CAD build for the part. Positions are in the model's coordinates, mm. Round coordinates to 2 decimals unless told otherwise and drop trailing zeros. Order: outer loops, then holes, each group sorted by start corner. A loop starts at its lowest first (then second) coordinate and runs counter-clockwise, first axis right, second up. Notation, with made-up numbers: (82.5, -11) -> (117.5, -11) arc R24 ccw to (117.5, 25) -> close; hole circle Ø8 at (23.5, 77). An arc over 180 degrees is marked (long way). Return JSON: item names as keys, results as strings. Group by question number.
Q1. Flat gauge pins, fed straight in: pin 1 (4 mm diameter, centred on y = -3, z = -8, fed in from +X); pin 2 (5 mm diameter, centred on y = -1, z = 7, fed in from -X); pin 3 (8 mm diameter, centred on y = -2, z = -3, fed in from +X). Where does each tip first touch, or does it go through?
Q2. Cut at C-C (x = 439). Write the cut outline in (y, z), then the cut area to 3 significant figures.
Q3. Cut at A-A (y = 3.5). Write the cut outline in (x, z), then the cut area to 3 significant figures.
Q4. Probe line 1 along Y through (x, z) = (187.5, -6.75); line 2 along X through (y, z) = (9.25, -2.5). List the from-to ranges inside material, lowest first.
Q5. Cut at B-B (z = -1.75). Write the cut outline in (x, y), then the cut area to 3 significant figures.
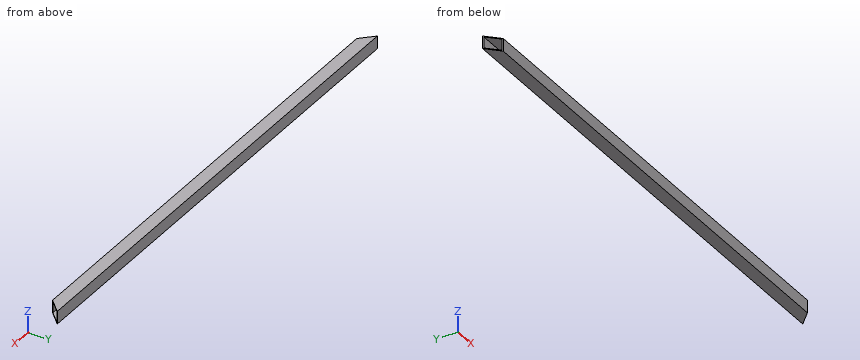
from build123d import *

# Parameters (mm, degrees)
SKETCH1_W               = 20
SKETCH1_H               = 20
SKETCH1_W_2             = 17.6
SKETCH1_H_2             = 17.6
BOSS_EXTRUDE1_DEPTH     = 800
CUT_EXTRUDE1_DEPTH      = 1
CUT_EXTRUDE1_DEPTH_BACK = 21
CUT_EXTRUDE2_DEPTH      = 1
CUT_EXTRUDE2_DEPTH_BACK = 21


with BuildPart() as part:
    # Sketch1 → Boss-Extrude1 (new body)
    with BuildSketch(Plane(origin=(0, 0, 0), x_dir=(0, 0, -1), z_dir=(1, 0, 0))):
        Rectangle(SKETCH1_W, SKETCH1_H)
        Rectangle(SKETCH1_W_2, SKETCH1_H_2, mode=Mode.SUBTRACT)
    extrude(amount=BOSS_EXTRUDE1_DEPTH)

    # Sketch2 → Cut-Extrude1 (cut, two sides)
    with BuildSketch(Plane.XY.offset(10)) as cut_extrude1_sk:
        Polygon((-1138.795415875, 1148.795415875), (0, 10), (20, -10), (1158.795415875, -1148.795415875), (-1118.795415875, -3426.386247626), (-3416.386247626, -1128.795415876), align=None)
    extrude(amount=CUT_EXTRUDE1_DEPTH, mode=Mode.SUBTRACT)
    extrude(cut_extrude1_sk.sketch, amount=-CUT_EXTRUDE1_DEPTH_BACK, mode=Mode.SUBTRACT)

    # Sketch3 → Cut-Extrude2 (cut, two sides)
    with BuildSketch(Plane.XY.offset(10)) as cut_extrude2_sk:
        Polygon((1938.795415875, 1148.795415875), (800, 10), (780, -10), (-358.795415875, -1148.795415875), (1918.795415876, -3426.386247626), (4216.386247626, -1128.795415875), align=None)
    extrude(amount=CUT_EXTRUDE2_DEPTH, mode=Mode.SUBTRACT)
    extrude(cut_extrude2_sk.sketch, amount=-CUT_EXTRUDE2_DEPTH_BACK, mode=Mode.SUBTRACT)


solid = part.part
Solution:
{
 "1": {"pin 1": "stops at x = 788.83", "pin 2": "stops at x = 9.27", "pin 3": "passes through"},
 "2": {"outline": "(-10, -10) -> (10, -10) -> (10, 10) -> (-10, 10) -> close; hole (-8.8, -8.8) -> (8.8, -8.8) -> (8.8, 8.8) -> (-8.8, 8.8) -> close", "area": "90.2 mm²"},
 "3": {"outline": "(6.5, -10) -> (793.5, -10) -> (793.5, -8.8) -> (6.5, -8.8) -> close; (6.5, 8.8) -> (793.5, 8.8) -> (793.5, 10) -> (6.5, 10) -> close", "area": "1,890 mm²"},
 "4": {"line 1": "y = -10 to -8.8, 8.8 to 10", "line 2": "x = 0.75 to 799.25"},
 "5": {"outline": "(0, 10) -> (1.2, 8.8) -> (798.8, 8.8) -> (800, 10) -> close; (18.8, -8.8) -> (20, -10) -> (780, -10) -> (781.2, -8.8) -> close", "area": "1,870 mm²"}
}
